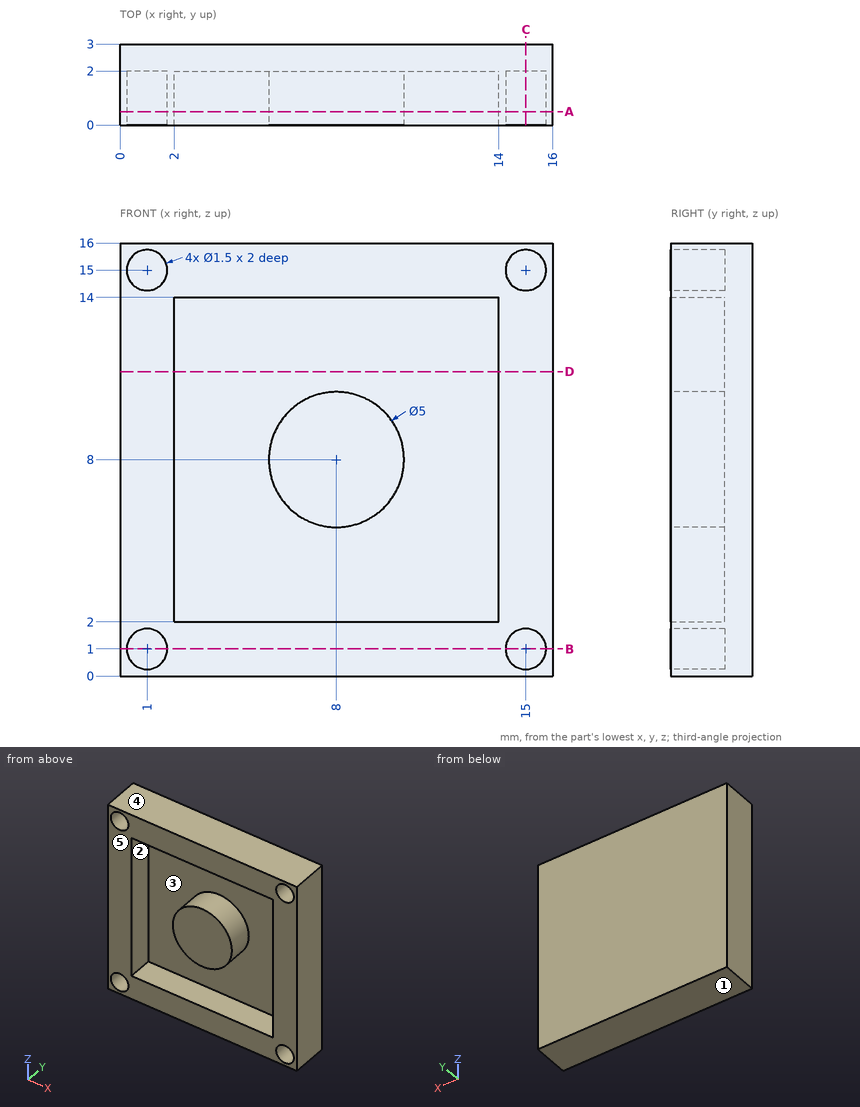
Input: dimensioned drawing with shaded views. Units: mm. Origin: part minimum x, y, z. A direction names the side the tool comes from. Coordinates: 2 decimals unless noted, no trailing zeros. Loops run counter-clockwise (first coordinate to the right, second up) from the corner with the lowest first, then second, coordinate; pieces in that order, holes last.
Q1. Set-up query: the marked faces 1 and 2. Return all of +Z, -Z, +X, -X, +Y, -Y with unobstructed straight access to the full face (end or side cutting, diameter ignored); none if empty.
Results are:
face 1: -Z, +X, -X, +Y, -Y
face 2: -Y
Q2. Mould query, pull axis Z, two halves, no side actions, for the marked faces 3, 4 and 5. Classes: +Z half, -Z half, draft (parallel to the pull), parting line (faces both ways), or undercut.
Results are:
face 3: undercut
face 4: +Z half
face 5: draft
Q3. Section D-D, the plane z = 11.25. Return the cut outline in (x, y).
Results are:
outline: (0, 0) - (2, 0) - (2, 2) - (14, 2) - (14, 0) - (16, 0) - (16, 3) - (0, 3) - close
Q4. Line query: line 1 along Z through (x, y) = (15, 1.65); line 2 along Z through (x, y) = (8, 1.85); line 3 along Z through (x, y) = (12.5, 0.2). Output: solid intervals per line, ascending.
Results are:
line 1: z = 0 to 0.25, 1.75 to 14.25, 15.75 to 16
line 2: z = 0 to 2, 5.5 to 10.5, 14 to 16
line 3: z = 0 to 2, 14 to 16
Q5. Contact query for a flat-ended pin moving along its axis: pin 1 (1.2 mm diameter, centred on x = 15, z = 1, fed in from -Y). Output: stop coordinate, or through.
Results are:
pin 1: stops at y = 2
Q6. Section B-B, the plane z = 1. Return the cut outline in (x, y).
Results are:
outline: (0, 0) - (0.25, 0) - (0.25, 2) - (1.75, 2) - (1.75, 0) - (14.25, 0) - (14.25, 2) - (15.75, 2) - (15.75, 0) - (16, 0) - (16, 3) - (0, 3) - close
Q7. Section C-C, the plane x = 15. Return the cut outline in (y, z), and give its area (3 significant figures).
Results are:
outline: (0, 0) - (3, 0) - (3, 16) - (0, 16) - (0, 15.75) - (2, 15.75) - (2, 14.25) - (0, 14.25) - (0, 1.75) - (2, 1.75) - (2, 0.25) - (0, 0.25) - close
area: 42.0 mm2
Q8. Section A-A, the plane y = 0.5. Return the cut outline in (x, z), and give its area (3 significant figures).
Results are:
outline: (0, 0) - (16, 0) - (16, 16) - (0, 16) - close; circle Ø5 at (8, 8); hole circle Ø1.5 at (1, 1); hole circle Ø1.5 at (1, 15); hole (2, 2) - (14, 2) - (14, 14) - (2, 14) - close; hole circle Ø1.5 at (15, 1); hole circle Ø1.5 at (15, 15)
area: 125 mm2
